Geometry: final body of the model. Coordinates: model frame, mm. A direction names the side the tool comes from. Give positions to 0.01 mm unless a question says otherwise; leave off trailing zeros.
Q1. Reachability of faces 1 (the face through (70, 0, -72)), 2 (the face through (62.98, 47.74, -66.95)), 3 (the face through (141.3, 27, -71)) from +Z, -Z, +X, -X, +Y, -Y: full face, straight path, thin tool, end or side. Return the list, or none.
Q2. Line query: L1, parallel to X at y = 48, z = -85 (3 decimals); L2, parallel to Z at x = 69.5, y = 5; L3, parallel to Y at x = 71.5, z = -66. Output: solid intervals per line, ascending.
Q3. Pin query (flat end, axial travel): pin 1 (4 mm diameter, centred on x = 70, y = 50.5, fed in from +Z); pin 2 (15 mm diameter, centred on x = 72, z = -79.5, fed in from +Y); pin 3 (2 mm diameter, centred on x = 73.5, y = 8.5, fed in from -Z). Return the tip coordinate at first contact, or that it passes through.
Q4. Draft query along X for faces 4 (the face through (1.5, 27, -71)), 5 (the face through (71, 27, -141.3)), 6 (the face through (70, 54, -88)), 7 (the face through (71, 48, -63.463)). Return one class per face: pulls with the +X half, pulls with the -X half, needs draft (parallel to the pull), parting line crosses it, or undercut.
```python
from build123d import *

# Parameters (mm, degrees)
SKETCH1_W           = 142.8
SKETCH1_H           = 142.8
BOSS_EXTRUDE1_DEPTH = 54
SKETCH2_W           = 10.53028371
SKETCH2_H           = 7.9375
CUT_EXTRUDE1_DEPTH  = 12.7
CUT_EXTRUDE5_DEPTH  = 55
CIRPATTERN3_COUNT   = 4


with BuildPart() as part:
    # Sketch1 → Boss-Extrude1 (new body)
    with BuildSketch(Plane(origin=(0, 0, 0), x_dir=(1, 0, 0), z_dir=(0, 1, 0))):
        with Locations((71.4, 71.4)):
            Rectangle(SKETCH1_W, SKETCH1_H)
    extrude(amount=BOSS_EXTRUDE1_DEPTH)

    # Sketch2 → Cut-Extrude1 (cut)
    with BuildSketch(Plane(origin=(0, 54, 0), x_dir=(1, 0, 0), z_dir=(0, 1, 0))):
        with BuildLine():
            ThreePointArc((76.665141855, 79.3375), (79.792737967, 75.904173), (80.925, 71.4))
            Line((80.925, 71.4), (80.925, 87.275))
            Line((80.925, 87.275), (61.875, 87.275))
            Line((61.875, 87.275), (61.875, 71.4))
            ThreePointArc((61.875, 71.4), (63.007262033, 75.904173), (66.134858145, 79.3375))
            ThreePointArc((66.134858145, 79.3375), (71.4, 80.925), (76.665141855, 79.3375))
        make_face()
        with BuildLine():
            ThreePointArc((76.665141855, 63.4625), (79.792737967, 66.895827), (80.925, 71.4))
            Line((80.925, 71.4), (76.665141855, 71.4))
            Line((76.665141855, 71.4), (76.665141855, 63.4625))
        make_face()
        with BuildLine():
            Line((76.665141855, 71.4), (80.925, 71.4))
            ThreePointArc((80.925, 71.4), (79.792737967, 75.904173), (76.665141855, 79.3375))
            Line((76.665141855, 79.3375), (76.665141855, 71.4))
        make_face()
        with BuildLine():
            Line((66.134858145, 63.4625), (66.134858145, 71.4))
            Line((66.134858145, 71.4), (61.875, 71.4))
            ThreePointArc((61.875, 71.4), (63.007262033, 66.895827), (66.134858145, 63.4625))
        make_face()
        with BuildLine():
            Line((61.875, 71.4), (66.134858145, 71.4))
            Line((66.134858145, 71.4), (66.134858145, 79.3375))
            ThreePointArc((66.134858145, 79.3375), (63.007262033, 75.904173), (61.875, 71.4))
        make_face()
        with Locations((71.4, 75.36875)):
            Rectangle(SKETCH2_W, SKETCH2_H)
        with BuildLine():
            Line((66.134858145, 79.3375), (76.665141855, 79.3375))
            ThreePointArc((76.665141855, 79.3375), (71.4, 80.925), (66.134858145, 79.3375))
        make_face()
        with Locations((71.4, 67.43125)):
            Rectangle(SKETCH2_W, SKETCH2_H)
    extrude(amount=-CUT_EXTRUDE1_DEPTH, mode=Mode.SUBTRACT)

    # Sketch7 → Cut-Extrude5 (cut, through all)
    with BuildSketch(Plane.XZ):
        Polygon((71.4, -142.8), (74.9, -142.8), (74.9, -141.3), (71.4, -141.3), (67.9, -141.3), (67.9, -142.8), align=None)
    cut_extrude5 = extrude(amount=-CUT_EXTRUDE5_DEPTH, mode=Mode.SUBTRACT)

    # CirPattern3: Cut-Extrude5 ×4 about axis
    cirpattern3_axis = Axis((71.4, 0, -71.4), (0, 1, 0))
    for i in range(1, CIRPATTERN3_COUNT):
        add(cut_extrude5.rotate(cirpattern3_axis, i * 360 / CIRPATTERN3_COUNT), mode=Mode.SUBTRACT)


solid = part.part
```
Data:
1. face 1: +Z, -Z, +X, -X, -Y
1. face 2: +Y
1. face 3: +X, +Y, -Y
2. L1: x = 0 to 61.875, 80.925 to 142.8
2. L2: z = -141.3 to -1.5
2. L3: y = 0 to 41.3
3. pin 1: stops at z = -1.5
3. pin 2: stops at y = 41.3
3. pin 3: stops at z = -141.3
4. face 4: pulls with the -X half
4. face 5: undercut
4. face 6: needs draft
4. face 7: undercut
